Autodesk Inventor part; units mm, degrees
ref_plane "YZ Plane" through (0, 0, 0) normal (1, 0, 0) x (0, 1, 0)
ref_plane "XZ Plane" through (0, 0, 0) normal (0, 1, 0) x (-1, 0, 0)
ref_plane "XY Plane" through (0, 0, 0) normal (0, 0, 1) x (1, 0, 0)
sketch "Szkic1" plane through (0, 0, 0) normal (0, 1, 0) x (-1, 0, 0)
  line L0 (0, 0) -> (102.05, 0)
  line L1 (102.05, 0) -> (102.05, 178.85)
  line L2 (102.05, 178.85) -> (0, 178.85)
  line L3 (0, 178.85) -> (0, 0)
  dimension "d0" = 178.85
  dimension "d1" = 102.05
extrude "Wyciągnięcie proste1" add sketch "Szkic1" along normal blind 17.75
sketch "Szkic2" plane through (0, 17.75, 0) normal (0, 1, 0) x (1, 0, 0)
  line L0 (-98.1, -3.35) -> (-3.95, -3.35)
  line L1 (-3.95, -3.35) -> (-3.95, -175.5)
  line L2 (-3.95, -175.5) -> (-98.1, -175.5)
  line L3 (-98.1, -175.5) -> (-98.1, -3.35)
  line L4 (-102.05, -178.85) -> (0, -178.85)
  line L5 (0, 0) -> (-102.05, 0)
  line L6 (-102.05, 0) -> (-102.05, -178.85)
  line L7 (0, -178.85) -> (0, 0)
  dimension "d4" = 3.35
  dimension "d5" = 3.35
  dimension "d6" = 3.95
  dimension "d7" = 3.95
extrude "Wyciągnięcie proste2" cut sketch "Szkic2" against normal blind 14.35 contours L0 L1 L2 L3
sketch "Szkic3" plane through (0, 3.4, 0) normal (0, 1, 0) x (1, 0, 0)
  circle A0 centre (-9.4, -9.45) radius 4.375
  circle A1 centre (-92.65, -9.45) radius 4.375
  circle A2 centre (-92.5, -63.1) radius 3
  circle A3 centre (-9.3, -62.65) radius 3
  circle A4 centre (-92.4, -115.4999) radius 3
  circle A5 centre (-9.05, -115.7994) radius 3
  circle A6 centre (-92.35, -169.9) radius 4.375
  circle A7 centre (-8.9504, -170.15) radius 4.375
  line L0 (-102.05, 0) -> (-102.05, -178.85)
  line L1 (0, 0) -> (-102.05, 0)
  line L2 (0, -178.85) -> (0, 0)
  line L3 (-98.1, -175.5) -> (-98.1, -3.35)
  line L4 (-3.95, -3.35) -> (-3.95, -175.5)
  dimension "d10" = 8.75
  dimension "d11" = 8.75
  dimension "d12" = 6
  dimension "d13" = 6
  dimension "d14" = 6
  dimension "d15" = 6
  dimension "d16" = 8.75
  dimension "d17" = 8.75
  dimension "d18" = 9.4
  dimension "d19" = 9.45
  dimension "d20" = 9.45
  dimension "d21" = 9.4
  dimension "d23" = 63.1
  dimension "d25" = 62.65
  dimension "d27" = 52.4
  dimension "d29" = 53.15
  dimension "d30" = 83.2
  dimension "d31" = 102.05
  dimension "d32" = 9.55
  dimension "d33" = 9.65
  dimension "d34" = 83.35
  dimension "d35" = 83.4
  dimension "d36" = 9.7
  dimension "d37" = 160.45
  dimension "d38" = 160.7
extrude "Wyciągnięcie proste3" add sketch "Szkic3" along normal blind 12 contours A0 | A1 | A6 | A7
sketch "Szkic4" plane through (-0.0028, 3.4, -0.0047) normal (0, 1, 0) x (1, 0, 0)
  circle A0 centre (-9.4, -9.45) radius 4.375
  circle A1 centre (-92.65, -9.45) radius 4.375
  circle A2 centre (-92.5, -63.1) radius 3
  circle A3 centre (-9.3, -62.65) radius 3
  circle A4 centre (-92.4, -115.4999) radius 3
  circle A5 centre (-9.05, -115.7994) radius 3
  circle A6 centre (-92.35, -169.9) radius 4.375
  circle A7 centre (-8.9504, -170.15) radius 4.375
  line L0 (-102.05, 0) -> (-102.05, -178.85)
  line L1 (0, 0) -> (-102.05, 0)
  line L2 (0, -178.85) -> (0, 0)
  line L3 (-98.1, -175.5) -> (-98.1, -3.35)
  line L4 (-3.95, -3.35) -> (-3.95, -175.5)
  dimension "d59" = 8.75
  dimension "d62" = 8.75
  dimension "d56" = 6
  dimension "d53" = 6
  dimension "d47" = 6
  dimension "d50" = 6
  dimension "d44" = 8.75
  dimension "d41" = 8.75
  dimension "d61" = 9.4
  dimension "d60" = 9.45
  dimension "d64" = 9.45
  dimension "d63" = 9.4
  dimension "d58" = 63.1
  dimension "d55" = 62.65
  dimension "d52" = 52.4
  dimension "d49" = 53.15
  dimension "d54" = 83.2
  dimension "d68" = 102.05
  dimension "d57" = 9.55
  dimension "d51" = 9.65
  dimension "d48" = 83.35
  dimension "d43" = 83.4
  dimension "d46" = 9.7
  dimension "d45" = 160.45
  dimension "d42" = 160.7
extrude "Wyciągnięcie proste4" add sketch "Szkic4" along normal blind 4.9 contours A2 | A3 | A4 | A5
sketch "Szkic5" plane through (-92.65, 15.4, 9.45) normal (0, 1, 0) x (1, 0, 0)
  circle A0 centre (0, 0) radius 1.975
  circle A1 centre (83.25, 0) radius 4.375
  circle A2 centre (83.25, 0) radius 1.975
  circle A3 centre (0.1472, -53.6453) radius 3
  circle A4 centre (0.1472, -53.6453) radius 1.2
  circle A5 centre (83.3472, -53.1953) radius 3
  circle A6 centre (83.3472, -53.1953) radius 1.2
  circle A7 centre (0.2472, -106.0452) radius 3
  circle A8 centre (0.2472, -106.0452) radius 1.2
  circle A9 centre (83.5972, -106.3447) radius 3
  circle A10 centre (83.5972, -106.3447) radius 1.2
  circle A11 centre (0.3, -160.45) radius 4.375
  circle A12 centre (0.3, -160.45) radius 1.975
  circle A13 centre (83.6996, -160.7) radius 4.375
  circle A14 centre (83.6996, -160.7) radius 1.975
  point P0 (92.65, 9.45)
  dimension "d69" = 3.95
  dimension "d70" = 3.95
  dimension "d71" = 2.4
  dimension "d72" = 2.4
  dimension "d73" = 2.4
  dimension "d74" = 2.4
  dimension "d75" = 3.95
  dimension "d76" = 3.95
extrude "Wyciągnięcie proste5" cut sketch "Szkic5" against normal through all contours A0 | A2 | A4 | A6 | A8 | A10 | A12 | A14
sketch "Szkic6" plane through (-98.1, 17.75, 175.5) normal (1, 0, 0) x (0, 0, -1)
  line L0 (144.273, -4.35) -> (156.273, -4.35)
  line L1 (156.273, -4.35) -> (156.273, -14.35)
  line L2 (156.273, -14.35) -> (144.273, -14.35)
  line L3 (144.273, -14.35) -> (144.273, -4.35)
  line L4 (0, -14.35) -> (172.15, -14.35)
  point P0 (175.5, -17.75)
  dimension "d79" = 10
  dimension "d80" = 12
extrude "Wyciągnięcie proste6" cut sketch "Szkic6" along normal through all both and the other way through all
sketch "Szkic7" plane through (-102.05, 0, 0) normal (-1, 0, 0) x (0, 0, 1)
  circle A0 centre (155.3753, 8.4) radius 3
  line L0 (19.227, 3.4) -> (19.227, 13.4)
  point P0 (0, 0)
  point P1 (19.227, 8.4)
  dimension "d83" = 6
extrude "Wyciągnięcie proste7" cut sketch "Szkic7" along normal through all both and the other way through all
properties part number "pudelko dol"
Source: CAD feature listing. Evaluate the final solid. Frame: model axes, mm. A direction names the side the tool comes from. Round coordinates to 2 decimals unless told otherwise and drop trailing zeros. Write each loop counter-clockwise with the first axis right and the second up, starting at its lowest first coordinate (ties: lowest second). Pieces come first, ordered by that corner, then holes. Notation, with made-up numbers: M 79.5,46.5 L 136.5,46.5 A13 cw 136.5,60.5 Z; hole C 14,40 d1. An arc over 180 degrees is marked long. Answer as a JSON object with one key per item and string values. Group by question number.
(1) Section query B-B on x = -59. Output: boundary loops of the cut face in (y, z), then the cut area to 3 significant figures.
(2) Mould query, pull axis Y, two halves, no side actions, for faces 1 (the flat face through (-9, 8.3, 64)), 2 (the cylindrical face through (-92.89, 5.82, 66.07)), 3 (the flat face through (-50, 0, 91)), 4 (the flat face through (-100, 8, 19.227)). Classes: +Y half, -Y half, draft (parallel to the pull), parting line (faces both ways), or undercut.
(3) First-contact query: pin 1 (2.5 mm diameter, centred on x = -94, z = 170, fed in from +Y); pin 2 (1.5 mm diameter, centred on x = -75, z = 54.5, fed in from -Y); pin 3 (1.4 mm diameter, centred on x = -9.05, z = 115.79, fed in from -Y); pin 4 (3 mm diameter, centred on x = -92.5, z = 63.1, fed in from +Y). Flat tips, straight axial feed; report the tip coordinate or a pass-through.
(4) Section query C-C on z = 73. Output: boundary loops of the cut face in (x, y).
(5) Section query A-A on z = 9.45. Output: boundary loops of the cut face in (x, y) (3 decimals).
(6) Reachability of faces 5 (the cylindrical face through (-9.208, 7.808, 168.192)), 6 (the flat face through (-2, 8, 31.227)), 7 (the flat face through (-91, 8.3, 115)) from +Z, -Z, +X, -X, +Y, -Y: full face, straight path, thin tool, end or side. Return the list, or none.
(7) Ray query, line 1 (Z direction, x = -10.5, y = 16.75); line 2 (X direction, y = 12.5, z = 53); line 3 (X direction, y = 12.75, z = 9). Return the intervals inside material, ascending. Write a range as [from, to].
Computed values:
{
 "1": {"outline": "M 0,0 L 17.75,0 L 17.75,3.35 L 3.4,3.35 L 3.4,175.5 L 17.75,175.5 L 17.75,178.85 L 0,178.85 Z", "area": "704 mm^2"},
 "2": {"face 1": "+Y half", "face 2": "draft", "face 3": "-Y half", "face 4": "undercut"},
 "3": {"pin 1": "y = 15.4", "pin 2": "y = 0", "pin 3": "through", "pin 4": "y = 8.3"},
 "4": {"outline": "M -102.05,0 L 0,0 L 0,17.75 L -3.95,17.75 L -3.95,3.4 L -98.1,3.4 L -98.1,17.75 L -102.05,17.75 Z"},
 "5": {"outline": "M -102.05,0 L -94.625,0 L -94.625,15.4 L -97.025,15.4 L -97.025,3.4 L -98.1,3.4 L -98.1,17.75 L -102.05,17.75 Z; M -90.675,0 L -11.375,0 L -11.375,15.4 L -13.775,15.4 L -13.775,3.4 L -88.275,3.4 L -88.275,15.4 L -90.675,15.4 Z; M -7.425,0 L 0,0 L 0,17.75 L -3.95,17.75 L -3.95,3.4 L -5.025,3.4 L -5.025,15.4 L -7.425,15.4 Z"},
 "6": {"face 5": "+Y, -Y", "face 6": "+X, -X", "face 7": "+Y"},
 "7": {"line 1": "[0, 3.35], [175.5, 178.85]", "line 2": "[-102.05, -98.1], [-3.95, 0]", "line 3": "[-102.05, -98.1], [-97, -94.57], [-90.73, -88.3], [-13.75, -11.32], [-7.48, -5.05], [-3.95, 0]"}
}
